Study the drawing (mm; zero at the part's minimum x, y, z) and answer. A direction names the side the tool comes from. Round coordinates to 2 decimals unless told otherwise and drop trailing zeros. Write each loop counter-clockwise with the first axis right and the second up, starting at its lowest first coordinate (ties: lowest second). Pieces come first, ordered by that corner, then holes. Notation, with made-up numbers: (77.25, 41) -> (96.25, 41) arc R11 cw to (96.25, 50) -> close; hole circle Ø1 at (61, 46.25). An arc over 180 degrees is marked (long way). Return JSON: item names as keys, results as strings.
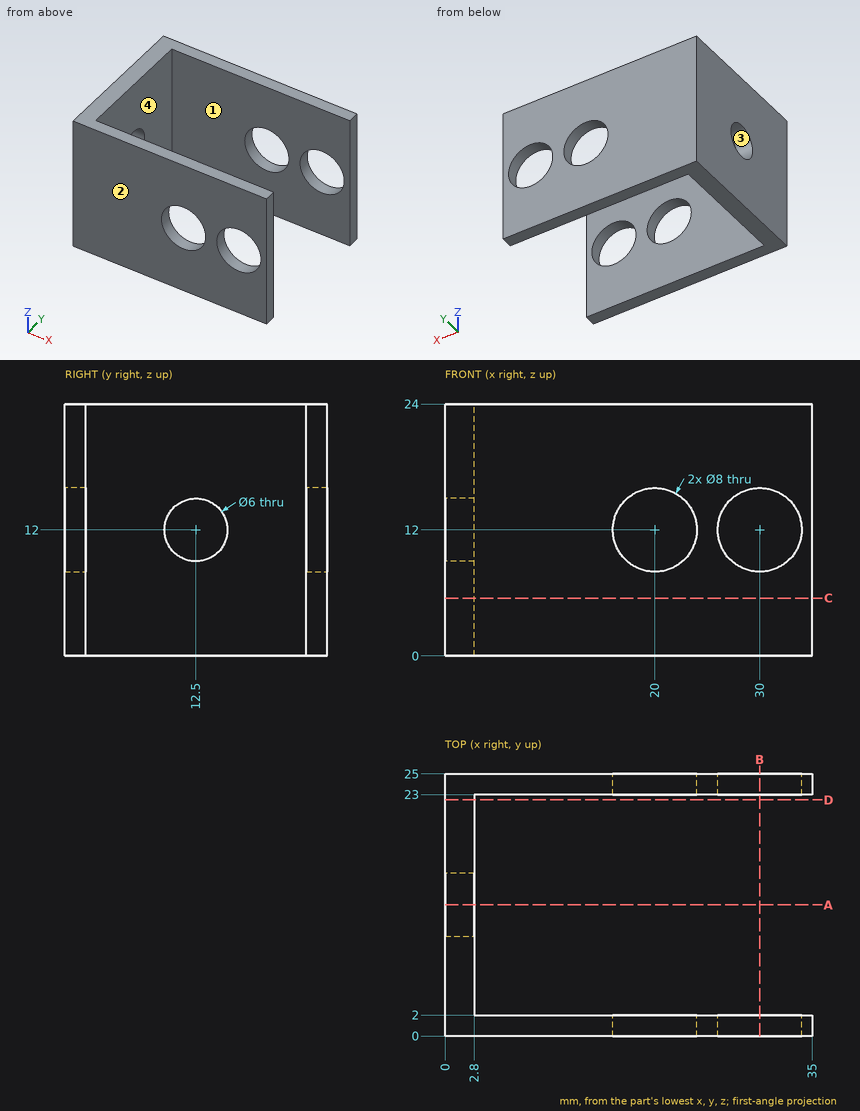
Item 1: Straight lines are drawn through the part: L1, parallel to X at y = 1.35, z = 12; L2, parallel to Y at x = 20.5, z = 4.5; L3, parallel to Z at x = 1.85, y = 12.5. For each, find the intervals that lie inside material, in ascending order. Write a range as [from, to].
Worked answers:
{"L1": "x = [0, 16], [24, 26], [34, 35]", "L2": "y = [0, 2], [23, 25]", "L3": "z = [0, 9], [15, 24]"}
Item 2: Section A-A (y = 12.5) is taken. Give the vertices of the cut face in (x, z).
Worked answers:
{"outline": "(0, 0) -> (2.8, 0) -> (2.8, 9) -> (0, 9) -> close; (0, 15) -> (2.8, 15) -> (2.8, 24) -> (0, 24) -> close"}
Item 3: A tool of negligible diameter and unlimited length cuts with its end or side. For the marked faces 1 and 2, from which of +Z, -Z, +X, -X, +Y, -Y can it reach the whole face along a straight path? Write none if from no direction.
Worked answers:
{"face 1": "+Z, -Z, +X", "face 2": "+Z, -Z, +X, -X, -Y"}
Item 4: A flat-ended cylindrical pin translates along its axis: pin 1 (4 mm diameter, centred on y = 15.5, z = 8, fed in from +X). Find the tip coordinate at first contact, or state that the pin passes through.
Worked answers:
{"pin 1": "stops at x = 2.8"}
Item 5: Section D-D (y = 22.5) is taken. Give the vertices of the cut face in (x, z), then the cut area to 3 significant figures.
Worked answers:
{"outline": "(0, 0) -> (2.8, 0) -> (2.8, 24) -> (0, 24) -> close", "area": "67.2 mm2"}
Item 6: Section B-B (x = 30) is taken. Give the vertices of the cut face in (y, z).
Worked answers:
{"outline": "(0, 0) -> (2, 0) -> (2, 8) -> (0, 8) -> close; (0, 16) -> (2, 16) -> (2, 24) -> (0, 24) -> close; (23, 0) -> (25, 0) -> (25, 8) -> (23, 8) -> close; (23, 16) -> (25, 16) -> (25, 24) -> (23, 24) -> close"}
Item 7: Section C-C (z = 5.5) is taken. Give the vertices of the cut face in (x, y).
Worked answers:
{"outline": "(0, 0) -> (35, 0) -> (35, 2) -> (2.8, 2) -> (2.8, 23) -> (35, 23) -> (35, 25) -> (0, 25) -> close"}
Item 8: For a pull along Z with two mould halves and no side action, classify the marked faces 3 and 4 as released by +Z, released by -Z, zero draft, split by the parting line, or undercut.
Worked answers:
{"face 3": "undercut", "face 4": "zero draft"}
